Input: part model. Units: mm. Frame: model coordinates. Coordinates: 2 decimals unless noted, no trailing zeros. Order: outer loops, then holes, each group sorted by start corner. A loop starts at its lowest first (then second) coordinate and runs counter-clockwise, first axis right, second up. Notation, with made-up numbers: M 77.25,69 L 134.25,69 A28 cw 134.25,87 Z; hole C 47.5,6.5 d2. An arc over 180 degrees is marked long. One line per item, written item: value.
Autodesk Inventor part; units mm, degrees
ref_plane "YZ Plane" through (0, 0, 0) normal (1, 0, 0) x (0, 1, 0)
ref_plane "XZ Plane" through (0, 0, 0) normal (0, 1, 0) x (-1, 0, 0)
ref_plane "XY Plane" through (0, 0, 0) normal (0, 0, 1) x (1, 0, 0)
sketch "Skizze1" plane through (0, 0, 0) normal (0, 0, 1) x (1, 0, 0)
  line L0 (-10.25, -8.8) -> (10.25, -8.8)
  line L1 (10.25, -8.8) -> (10.25, 8.8)
  line L2 (10.25, 8.8) -> (-10.25, 8.8)
  line L3 (-10.25, 8.8) -> (-10.25, -8.8)
  line L4 (-10.25, -8.8) -> (10.25, 8.8) construction
  line L5 (10.25, -8.8) -> (-10.25, 8.8) construction
  point P0 (0, 0)
  dimension "d0" = 20.5
  dimension "d1" = 17.6
extrude "Extrusion1" add sketch "Skizze1" along normal blind 0.75
fillet "Rundung1" radius 3 4 edges at (10.25, -8.8, 0.375) (-10.25, -8.8, 0.375) (-10.25, 8.8, 0.375) (10.25, 8.8, 0.375)
sketch "Skizze2" plane through (0, 0, 0.75) normal (0, 0, 1) x (1, 0, 0)
  line L0 (7.75, -6.05) -> (-7.75, -6.05) construction
  line L1 (-7.75, -6.05) -> (-7.75, 6.05) construction
  line L2 (-7.75, 6.05) -> (7.75, 6.05) construction
  line L3 (7.75, 6.05) -> (7.75, -6.05) construction
  line L4 (7.75, -6.05) -> (-7.75, 6.05) construction
  line L5 (-7.75, -6.05) -> (7.75, 6.05) construction
  circle A0 centre (-7.75, -6.05) radius 1.25
  circle A1 centre (7.75, -6.05) radius 1.25
  line L6 (-15.2198, 0) -> (15.2198, 0) construction
  circle A2 centre (0, 6.05) radius 0.5
  line L7 (-5.21, 6.05) -> (10.29, 6.05) construction
  circle A3 centre (2.54, 6.05) radius 0.5
  line L8 (-2.67, 6.05) -> (12.83, 6.05) construction
  circle A4 centre (5.08, 6.05) radius 0.5
  line L9 (-0.13, 6.05) -> (15.37, 6.05) construction
  circle A5 centre (7.62, 6.05) radius 0.5
  line L10 (-10.29, 6.05) -> (5.21, 6.05) construction
  circle A6 centre (-2.54, 6.05) radius 0.5
  line L11 (-7.75, 6.05) -> (7.75, 6.05) construction
  circle A7 centre (0, 6.05) radius 0.5
  line L12 (-5.21, 6.05) -> (10.29, 6.05) construction
  circle A8 centre (2.54, 6.05) radius 0.5
  line L13 (-2.67, 6.05) -> (12.83, 6.05) construction
  circle A9 centre (5.08, 6.05) radius 0.5
  line L14 (-12.83, 6.05) -> (2.67, 6.05) construction
  circle A10 centre (-5.08, 6.05) radius 0.5
  line L15 (-10.29, 6.05) -> (5.21, 6.05) construction
  circle A11 centre (-2.54, 6.05) radius 0.5
  line L16 (-7.75, 6.05) -> (7.75, 6.05) construction
  circle A12 centre (0, 6.05) radius 0.5
  line L17 (-5.21, 6.05) -> (10.29, 6.05) construction
  circle A13 centre (2.54, 6.05) radius 0.5
  line L18 (-15.37, 6.05) -> (0.13, 6.05) construction
  circle A14 centre (-7.62, 6.05) radius 0.5
  line L19 (-12.83, 6.05) -> (2.67, 6.05) construction
  circle A15 centre (-5.08, 6.05) radius 0.5
  line L20 (-10.29, 6.05) -> (5.21, 6.05) construction
  circle A16 centre (-2.54, 6.05) radius 0.5
  line L21 (-7.75, 6.05) -> (7.75, 6.05) construction
  circle A17 centre (0, 6.05) radius 0.5
  point P0 (0, 0)
  dimension "d5" = 15.5
  dimension "d6" = 12.1
  dimension "d7" = 2.5
  dimension "d10" = 1
  dimension "d13" = 2.54
  dimension "d16" = 2.54
extrude "Extrusion2" cut sketch "Skizze2" against normal through all
sketch "Skizze3" plane through (0, 0, 0.75) normal (0, 0, 1) x (1, 0, 0)
  line L0 (-1.45, -3.9) -> (1.45, -3.9)
  line L1 (1.45, -3.9) -> (1.45, 1.3)
  line L2 (1.45, 1.3) -> (-1.45, 1.3)
  line L3 (-1.45, 1.3) -> (-1.45, -3.9)
  line L4 (-1.45, -3.9) -> (1.45, 1.3) construction
  line L5 (1.45, -3.9) -> (-1.45, 1.3) construction
  line L6 (0, -13.1898) -> (0, 13.1898) construction
  circle A0 centre (0, -2.8) radius 0.25
  circle A1 centre (0, 0.7) radius 0.25
  line L7 (-15.2198, 0) -> (15.2198, 0) construction
  point P0 (0, 0)
  point P1 (0, -1.3)
  point P2 (0, -1.3)
  dimension "d21" = 2.9
  dimension "d22" = 5.2
  dimension "d23" = 0.5
  dimension "d24" = 0.5
  dimension "d25" = 0.6
  dimension "d26" = 1.1
  dimension "d27" = 1.3
extrude "Extrusion3" add sketch "Skizze3" along normal blind 1
properties part number "VL6180X-Time_of_Flight_Sensor"
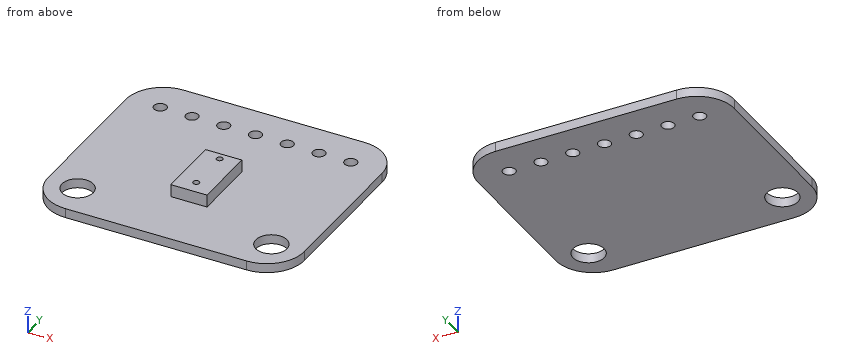
(1) Cut plane A-A on x = 5.08. Output: boundary loops of the cut face in (y, z).
Data:
outline: M -8.8,0 L 5.55,0 L 5.55,0.75 L -8.8,0.75 Z; M 6.55,0 L 8.8,0 L 8.8,0.75 L 6.55,0.75 Z
(2) Cut plane B-B on z = 1.25. Output: boundary loops of the cut face in (x, y).
Data:
outline: M -1.45,-3.9 L 1.45,-3.9 L 1.45,1.3 L -1.45,1.3 Z; hole C 0,-2.8 d0.5; hole C 0,0.7 d0.5
(3) Cut plane C-C on y = 0.7. Output: boundary loops of the cut face in (x, z).
Data:
outline: M -10.25,0 L 10.25,0 L 10.25,0.75 L 1.45,0.75 L 1.45,1.75 L 0.25,1.75 L 0.25,0.75 L -0.25,0.75 L -0.25,1.75 L -1.45,1.75 L -1.45,0.75 L -10.25,0.75 Z
(4) Cut plane D-D on y = -6.05. Output: boundary loops of the cut face in (x, z).
Data:
outline: M -10.24,0 L -9,0 L -9,0.75 L -10.24,0.75 Z; M -6.5,0 L 6.5,0 L 6.5,0.75 L -6.5,0.75 Z; M 9,0 L 10.24,0 L 10.24,0.75 L 9,0.75 Z
(5) Ray query, line 1 (Y direction, x = 0, z = 1.5); line 2 (Y direction, x = -2.5, z = 0.5); line 3 (Z direction, x = -5.5, y = 2). Return the intervals inside material, ascending. Write a range as from..to.
Data:
line 1: y = -3.9..-3.05, -2.55..0.45, 0.95..1.3
line 2: y = -8.8..5.55, 6.55..8.8
line 3: z = 0..0.75
(6) First-contact query: pin 1 (1 mm diameter, centred on y = -4.5, z = 1.5, fed in from +X); pin 2 (3 mm diameter, centred on x = -7.75, y = -6.05, fed in from +Z). Flat tips, straight axial feed; report the tip coordinate or a pass-through.
Data:
pin 1: passes through
pin 2: stops at z = 0.75
